Design review of the part built by this model. Coordinates are the model's own, in mm. Face numbers are marked on the shaded views. A direction names the side the tool comes from. Round coordinates to 2 decimals unless told otherwise and drop trailing zeros. Answer as CSV lines item,"result". Start each with the question number.
(1) Wall thickness on L1, parallel to Y at x = 5.5, z = 0; L2, parallel to Z at x = 2, y = 1; L3, parallel to Z at x = 4, y = -27: over which ranges is each line inside the solid? List them lowest first.
(2) For the marked faces 4, 5 and 6, list the 3-axis set-ups (+Z, -Z, +X, -X, +Y, -Y) from which the entire face can be reached by the end or side of a thin tool; tool diameter is ignored.
(3) Mouldability with a two-part tool opening along Y and no side actions: class the marked faces 1, 2 and 3 as released by +Y, released by -Y, zero draft, split by the parting line, or undercut.
(4) For P1, Ø16, axis at y = -34, z = -4.5, coming from the +X side; P2, Ø4, axis at y = -44.99, z = -16.6, coming from the -X side; P3, Ø6, axis at y = 14, z = -13.5, coming from the +X side; P4, Ø2.5, axis at x = 2.5, y = -21, coming from the -Z side, all flat-tipped, find the tip position at first contact; note any pin that passes through.
from build123d import *
from build123d.topology import SkipClean

# Parameters (mm, degrees)
BOSS_EXTRUDE1_DEPTH                               = 7.6
BOSS_EXTRUDE1_DEPTH_BACK                          = 2
CUT_EXTRUDE1_DEPTH                                = 70.244569428
CUT_EXTRUDE1_DEPTH_BACK                           = 70.244569428
SKETCH9_R                                         = 20
SKETCH10_R                                        = 3.1
CUT_EXTRUDE2_DEPTH                                = 70.244569428
SKETCH11_R                                        = 26.7
CUT_EXTRUDE3_DEPTH                                = 70.244569428
CUT_EXTRUDE4_DEPTH                                = 70.244569428
CUT_EXTRUDE4_DEPTH_BACK                           = 70.244569428
SKETCH12_W                                        = 5.7
SKETCH12_H                                        = 2.4
CUT_EXTRUDE5_START                                = 28.174078
CUT_EXTRUDE5_DEPTH                                = 6
M4_CLEARANCE_HOLE1_D                              = 4.5
BOSS_EXTRUDE2_DEPTH                               = 4
CHAMFER1_SIZE                                     = 2
CHAMFER2_SIZE                                     = 0.8
CSK_FOR_M2_5_FLAT_HEAD_MACHINE_SCREW1_D           = 2.9
CSK_FOR_M2_5_FLAT_HEAD_MACHINE_SCREW1_CSINK_D     = 5.5
CSK_FOR_M2_5_FLAT_HEAD_MACHINE_SCREW1_CSINK_ANGLE = 90
CIRPATTERN1_COUNT                                 = 3
LPATTERN1_COUNT                                   = 2
LPATTERN1_PITCH                                   = 56
LPATTERN1_COPY_1_D                                = 2.9
LPATTERN1_COPY_1_CSINK_D                          = 5.5
LPATTERN1_COPY_1_CSINK_ANGLE                      = 90
LPATTERN1_COPY_2_D                                = 2.9
LPATTERN1_COPY_2_CSINK_D                          = 5.5
LPATTERN1_COPY_2_CSINK_ANGLE                      = 90


with BuildPart() as part:
    # Sketch2 → Boss-Extrude1 (new, two sides: drawn at the far end of the back side and taken through both)
    with BuildSketch(Plane.YZ.offset(-BOSS_EXTRUDE1_DEPTH_BACK)):
        with BuildLine():
            Line((-12.727922061, -32.553844327), (-14.317300295, -30.964466094))
            ThreePointArc((-14.317300295, -30.964466094), (-15.939417039, -29.880602337), (-17.852834201, -29.5))
            Line((-17.852834201, -29.5), (-28, -29.5))
            ThreePointArc((-28, -29.5), (-48.859650045, -20.859650045), (-57.5, 0))
            Line((-57.5, 0), (-57.5, 28.174077734))
            Line((-57.5, 28.174077734), (0, 28.174077734))
            Line((0, 28.174077734), (0, -37.825922266))
            ThreePointArc((0, -37.825922266), (-6.888301783, -36.455753851), (-12.727922061, -32.553844327))
        make_face()
    extrude(amount=BOSS_EXTRUDE1_DEPTH + BOSS_EXTRUDE1_DEPTH_BACK)

    # Sketch9 → Cut-Extrude1 (cut, two sides: drawn at the far end of the back side and taken through both)
    with BuildSketch(Plane.YZ.offset(-CUT_EXTRUDE1_DEPTH_BACK)):
        with Locations(Location((-28, 0, 0), (0, 0, 90))):
            Circle(SKETCH9_R)
    extrude(amount=CUT_EXTRUDE1_DEPTH + CUT_EXTRUDE1_DEPTH_BACK, mode=Mode.SUBTRACT)

    # Sketch10 → Cut-Extrude2 (cut, through all)
    with BuildSketch(Plane.YZ):
        with Locations((0, 16.174077734)):
            Circle(SKETCH10_R)
        with Locations(Location((-8.485281374, -28.31120364, 0), (0, 0, 270))):
            Circle(SKETCH10_R)
        with Locations((0, -31.825922266)):
            Circle(SKETCH10_R)
        with Locations((8.485281374, -28.31120364)):
            Circle(SKETCH10_R)
        with Locations(Location((-51, 21.674077734, 0), (0, 0, 270))):
            Circle(SKETCH10_R)
    extrude(amount=CUT_EXTRUDE2_DEPTH, mode=Mode.SUBTRACT)

    # Sketch11 → Cut-Extrude3 (cut, through all)
    with BuildSketch(Plane.YZ):
        with Locations(Location((-28, 0, 0), (0, 0, 270))):
            Circle(SKETCH11_R)
    extrude(amount=CUT_EXTRUDE3_DEPTH, mode=Mode.SUBTRACT)

    # Sketch12 → Cut-Extrude4 (cut, two sides: drawn at the far end of the back side and taken through both)
    with BuildSketch(Plane.YZ.offset(-CUT_EXTRUDE4_DEPTH_BACK)):
        with Locations((0, 24.974077734)):
            Rectangle(SKETCH12_W, SKETCH12_H)
    extrude(amount=CUT_EXTRUDE4_DEPTH + CUT_EXTRUDE4_DEPTH_BACK, mode=Mode.SUBTRACT)

    # Sketch13 → Cut-Extrude5 (cut)
    with BuildSketch(Plane.XY.offset(CUT_EXTRUDE5_START)):
        Polygon((2.5, -2.404163056), (4.904163056, 0), (2.5, 2.404163056), (0.095836944, 0), align=None)
    extrude(amount=-CUT_EXTRUDE5_DEPTH, mode=Mode.SUBTRACT)

    # M4 Clearance Hole1 (through all)
    with Locations(Plane.ZY.offset(2)):
        with Locations((16.174077734, 0), (-28.31120364, -8.485281374), (-31.825922266, 0), (21.674077734, -51)):
            Hole(M4_CLEARANCE_HOLE1_D / 2)

    # Sketch20 → Boss-Extrude2 (add)
    with BuildSketch(Plane.XY.offset(28.174077734)):
        Polygon((-2, -51.5), (-2, -57.5), (4, -57.5), (4, -55.5), (0, -51.5), align=None)
    extrude(amount=BOSS_EXTRUDE2_DEPTH)

    # Chamfer1
    chamfer1_edges = [part.edges().sort_by_distance(p)[0] for p in [
        (-2, -48.859650045, -20.859650045),
        (-2, -22.9264171, -29.5),
        (-2, -15.939417039, -29.880602337),
        (-2, -13.522611178, -31.759155211),
        (-2, -6.888301783, -36.455753851),
        (-2, -57.5, 16.087038867),
    ]]
    chamfer(chamfer1_edges, length=CHAMFER1_SIZE)

    # Chamfer2
    chamfer2_edges = [part.edges().sort_by_distance(p)[0] for p in [
        (7.6, -3.1, 16.174077734),
        (7.6, -3.1, -31.825922266),
        (7.6, -8.485281374, -25.21120364),
        (7.6, -51, 24.774077734),
    ]]
    chamfer(chamfer2_edges, length=CHAMFER2_SIZE)

    # Mirror1: part across plane


with BuildPart() as part_1:
    with SkipClean():  # the faces are left unmerged after this step: merging them gives an invalid solid
        add(part.part)
        add(part.part.mirror(Plane(origin=(0, 0, 0), x_dir=(0, 0, 1), z_dir=(0, -1, 0))))

    # CSK for M2.5 Flat Head Machine Screw1 (through all)
    with Locations(Plane.ZY.offset(2)):
        with Locations((23.011048917, -33.878275914)):
            csk_for_m2_5_flat_head_machine_screw1 = CounterSinkHole(CSK_FOR_M2_5_FLAT_HEAD_MACHINE_SCREW1_D / 2, CSK_FOR_M2_5_FLAT_HEAD_MACHINE_SCREW1_CSINK_D / 2, counter_sink_angle=CSK_FOR_M2_5_FLAT_HEAD_MACHINE_SCREW1_CSINK_ANGLE)

    # CirPattern1: CSK for M2.5 Flat Head Machine Screw1 ×3 about axis
    with SkipClean():  # the faces are left unmerged after this step: merging them gives an invalid solid
        cirpattern1_axis = Axis((0, -28, 0), (1, 0, 0))
        for i in range(1, CIRPATTERN1_COUNT):
            add(csk_for_m2_5_flat_head_machine_screw1.rotate(cirpattern1_axis, i * 360 / CIRPATTERN1_COUNT), mode=Mode.SUBTRACT)

    # LPattern1: CSK for M2.5 Flat Head Machine Screw1 ×2
    with SkipClean():  # the faces are left unmerged after this step: merging them gives an invalid solid
        with Locations(*[(0, i * LPATTERN1_PITCH, 0) for i in range(1, LPATTERN1_COUNT)]):
            add(csk_for_m2_5_flat_head_machine_screw1, mode=Mode.SUBTRACT)

    # LPattern1 copy 1 (through all)
    with Locations(Plane(origin=(-2, 14, 24.248711306), x_dir=(-6.7609180727612354e-15, -0.8660254037844387, -0.4999999999999998), z_dir=(-1, 0, 0))):
        with Locations((23.011048917, -33.878275914)):
            CounterSinkHole(LPATTERN1_COPY_1_D / 2, LPATTERN1_COPY_1_CSINK_D / 2, counter_sink_angle=LPATTERN1_COPY_1_CSINK_ANGLE)

    # LPattern1 copy 2 (through all)
    with Locations(Plane(origin=(-2, 14, -24.248711306), x_dir=(-6.7609180727612354e-15, 0.8660254037844384, -0.5000000000000004), z_dir=(-1, 0, 0))):
        with Locations((23.011048917, -33.878275914)):
            CounterSinkHole(LPATTERN1_COPY_2_D / 2, LPATTERN1_COPY_2_CSINK_D / 2, counter_sink_angle=LPATTERN1_COPY_2_CSINK_ANGLE)


solid = part_1.part
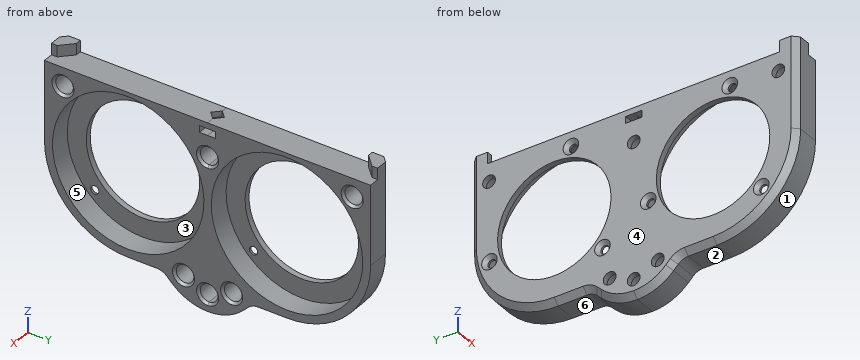
Determined:
1,L1,"y = -57.5 to -54.7, -1.3 to 1.3, 54.7 to 57.5"
1,L2,"z = -37.8 to -34.76, -28.89 to 13.24, 19.11 to 22.17"
1,L3,"z = -29.5 to -26.68, 26.68 to 28.17"
2,face 4,"+Z, -Z, -X, +Y, -Y"
2,face 5,"+X"
2,face 6,"-Z, +X, -X, +Y"
3,face 1,"released by -Y"
3,face 2,"zero draft"
3,face 3,"undercut"
4,P1,"passes through"
4,P2,"stops at x = -1.25"
4,P3,"stops at x = 0"
4,P4,"stops at z = -29.5"
